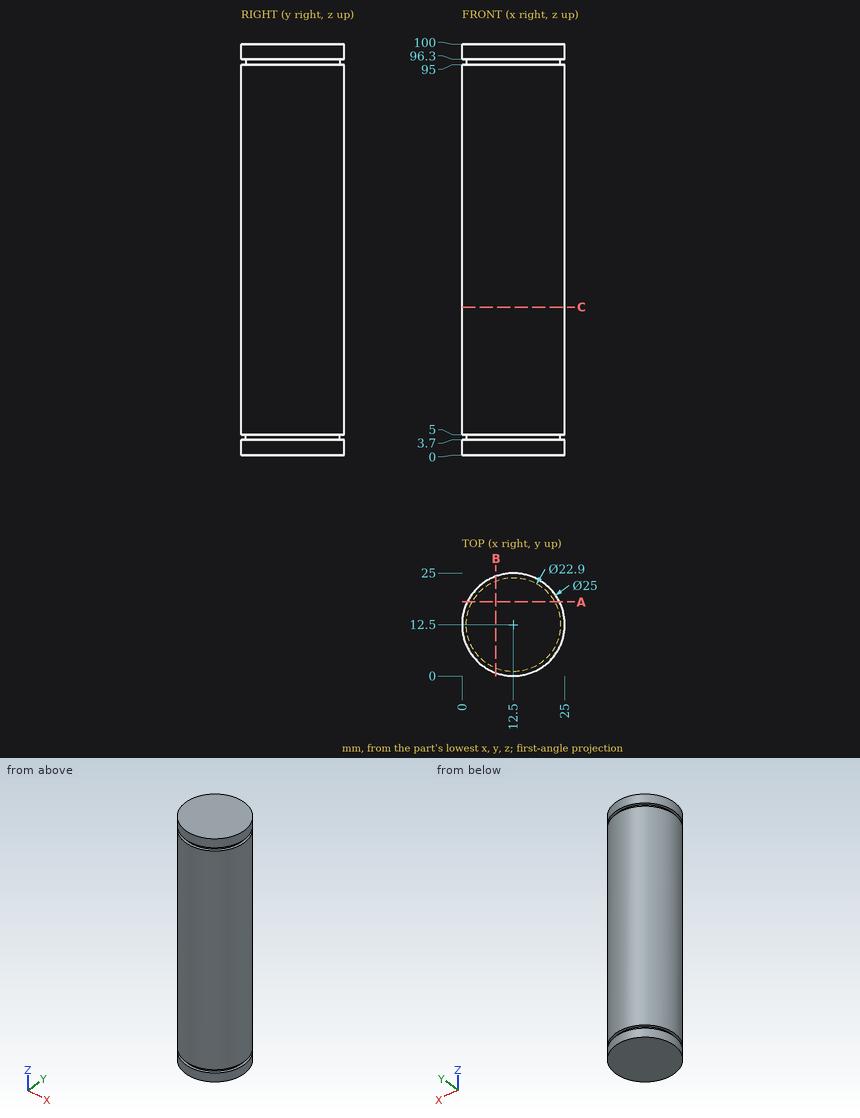
Here's the drawing with two shaded views (mm, measured from the low corner). I have some questions. Coordinates: 2 decimals unless noted, no trailing zeros. Order: outer loops, then holes, each group sorted by start corner. A loop starts at its lowest first (then second) coordinate and runs counter-clockwise, first axis right, second up.
Item 1: If we section it at A-A on y = 18: List the corners of the cut face in (x, z) for me, plus the area to 3 significant figures.
Result sheet:
outline: (1.28, 0) - (23.72, 0) - (23.72, 3.7) - (22.54, 3.7) - (22.54, 5) - (23.72, 5) - (23.72, 95) - (22.54, 95) - (22.54, 96.3) - (23.72, 96.3) - (23.72, 100) - (1.28, 100) - (1.28, 96.3) - (2.46, 96.3) - (2.46, 95) - (1.28, 95) - (1.28, 5) - (2.46, 5) - (2.46, 3.7) - (1.28, 3.7) - close
area: 2,240 mm2
Item 2: If we section it at B-B on x = 8.25: List the corners of the cut face in (y, z) for me, plus the area to 3 significant figures.
Result sheet:
outline: (0.74, 0) - (24.26, 0) - (24.26, 3.7) - (23.13, 3.7) - (23.13, 5) - (24.26, 5) - (24.26, 95) - (23.13, 95) - (23.13, 96.3) - (24.26, 96.3) - (24.26, 100) - (0.74, 100) - (0.74, 96.3) - (1.87, 96.3) - (1.87, 95) - (0.74, 95) - (0.74, 5) - (1.87, 5) - (1.87, 3.7) - (0.74, 3.7) - close
area: 2,350 mm2
Item 3: For P1, Ø3, axis at y = 21, z = 10, coming from the +X side; P2, Ø12, axis at y = 6, z = 87, coming from the +X side, each with a flat end and sliding along its axis, tell me the tip position at first contact or that it passes through.
Result sheet:
P1: stops at x = 22.86
P2: stops at x = 24.99
Item 4: I need wall thicknesses on line 1 (Z direction, x = 20, y = 22.25); line 2 (Y direction, x = 12, z = 51.5). Which ranges of each line are inside material? Lowest first, please.
Result sheet:
line 1: z = 0 to 3.7, 5 to 95, 96.3 to 100
line 2: y = 0.01 to 24.99
Item 5: If we section it at C-C on z = 36: List the corners of the cut face in (x, y) for me, plus the area to 3 significant figures.
Result sheet:
outline: circle Ø25 at (12.5, 12.5)
area: 491 mm2
